Verification items for the finished model (mm, model axes). Face numbers are marked on the shaded views. A direction names the side the tool comes from. Give positions to 0.01 mm unless a question says otherwise; leave off trailing zeros. Order: outer loops, then holes, each group sorted by start corner. A loop starts at its lowest first (then second) coordinate and runs counter-clockwise, first axis right, second up. Notation, with made-up numbers: (58, 38) - (110, 38) arc R24 cw to (110, 77) - close; hole circle Ø3 at (57.5, 65). An arc over 180 degrees is marked (long way). Answer as a JSON object with one key per item and string values.
```python
from build123d import *

# Parameters (mm, degrees)
RESSALTO_EXTRUS_O1_DEPTH = 11.849977
ESCALA1_SCALE            = 0.681818182


with BuildPart() as part:
    # Esboço1 → Ressalto-extrusão1 (new body)
    with BuildSketch(Plane.XY):
        with BuildLine():
            ThreePointArc((-10.685745363, -67.703603991), (-26.769323244, -33.991425444), (2.462180193, -10.738217779))
            Line((2.462180193, -10.738217779), (2.462180193, -0.672237217))
            Line((2.462180193, -0.672237217), (2.462180193, 19.360753065))
            ThreePointArc((2.462180193, 19.360753065), (-0.537819807, 22.360753065), (-3.537819807, 19.360753065))
            Line((-3.537819807, 19.360753065), (-3.478607435, 18.767652629))
            Line((-3.478607435, 18.767652629), (-0.816088481, -7.901455538))
            ThreePointArc((-0.816088481, -7.901455538), (-26.821074104, -25.523388901), (-26.291187743, -56.932162089))
            Line((-26.291187743, -56.932162089), (-31.663381791, -61.605561148))
            ThreePointArc((-31.663381791, -61.605561148), (-24.444874339, -70.335690922), (-15.068387215, -76.692066062))
            Line((-15.068387215, -76.692066062), (-10.685745363, -67.703603991))
        make_face()
    extrude(amount=RESSALTO_EXTRUS_O1_DEPTH)


with BuildPart() as part_1:
    # Escala1: scaled about (0, 0, 0)
    add(part.part.scale(ESCALA1_SCALE))


solid = part_1.part
```
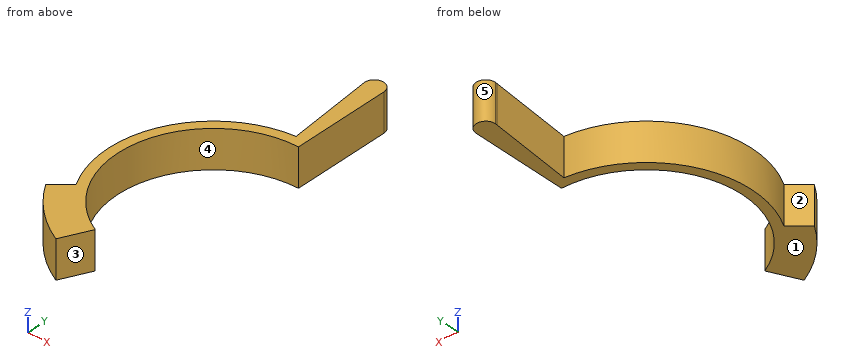
(1) Material ranges on line 1 along Y through (x, z) = (-8.5, 5); line 2 along Y through (x, z) = (-9, 4.5); line 3 along X through (y, z) = (-12, 7.25), recorded low to high. Write a range as [from, to].
Computed values:
{"line 1": "y = [-48.65, -45.52], [-10.03, -7.71]", "line 2": "y = [-49.68, -45.22], [-10.33, -7.97]", "line 3": "x = [-14.36, -11.34]"}
(2) Section check D-D (y = -37.5). Record the cut outline in (x, z).
Computed values:
{"outline": "(-18.61, 0) - (-16.32, 0) - (-16.32, 8.08) - (-18.61, 8.08) - close"}
(3) Section check A-A (x = -1.75). Record the cut outline in (y, z).
Computed values:
{"outline": "(-7.61, 0) - (-5.54, 0) - (-5.54, 8.08) - (-7.61, 8.08) - close; (6.57, 0) - (14.71, 0) - (14.71, 8.08) - (6.57, 8.08) - close"}
(4) Gauge pin test, flat ends, axial feed: pin 1 Ø3 at (x, z) = (-5, 4) entering from +Y; pin 2 Ø1 at (y, z) = (-11.5, 5.5) entering from +X. Record the tip position at first contact, or that the pin passes through.
Computed values:
{"pin 1": "stops at y = -5.88", "pin 2": "stops at x = -10.02"}
(5) Section check C-C (x = -11.25). Record the cut outline in (y, z), then the cut area to 3 significant figures.
Computed values:
{"outline": "(-51.79, 0) - (-43.63, 0) - (-43.63, 8.08) - (-51.79, 8.08) - close; (-11.93, 0) - (-9.36, 0) - (-9.36, 8.08) - (-11.93, 8.08) - close", "area": "86.7 mm²"}
(6) Access from +Z, -Z, +X, -X, +Y, -Y to the whole of each face (thin tool, end or side, straight path). Record for the marked faces 1 and 2.
Computed values:
{"face 1": "-Z, +X, -X, +Y, -Y", "face 2": "+Z, -Z, -X"}
(7) Release check for a two-part mould opening along Y. For the marked faces 3, 4 and 5 record: pulls with the +Y half, pulls with the -Y half, needs draft (parallel to the pull), parting line crosses it, or undercut.
Computed values:
{"face 3": "pulls with the -Y half", "face 4": "undercut", "face 5": "pulls with the +Y half"}
(8) Section check B-B (z = 2.25). Record the cut outline in (x, y), then the cut area to 3 significant figures.
Computed values:
{"outline": "(-21.59, -42) arc R27.27 ccw to (-10.27, -52.29) - (-7.29, -46.16) arc R20.45 cw to (1.68, -7.32) - (1.68, 13.2) arc R2.05 ccw to (-2.41, 13.2) - (-0.56, -5.39) arc R22.5 ccw to (-17.93, -38.82) - close", "area": "253 mm²"}
